Could you check a few things on this model? Use its own coordinates, in mm. Round coordinates to 2 decimals unless told otherwise and drop trailing zeros. Loops run counter-clockwise (first coordinate to the right, second up) from the corner with the lowest first, then second, coordinate; pieces in that order, holes last. Notation, with made-up numbers: (36.5, 39) - (82.5, 39) arc R19 ccw to (82.5, 70) - close; hole circle Ø4 at (74, -32.5). An arc over 180 degrees is marked (long way). Put each result on its own line as item: value. Start each with the question number.
from build123d import *

# Parameters (mm, degrees)
F0_R     = 10
F1_DEPTH = 2.5


with BuildPart() as f1:
    # F0 (on Front) → F1 (new body, symmetric)
    with BuildSketch(Plane.XZ):
        with BuildLine():
            ThreePointArc((0, 15), (10.606602, 10.606602), (15, 0))
            ThreePointArc((15, 0), (10.606602, -10.606602), (0, -15))
            Line((0, -15), (180, -15))
            ThreePointArc((180, -15), (165, 0), (180, 15))
            Line((180, 15), (0, 15))
        make_face()
        with BuildLine():
            ThreePointArc((0, -15), (10.606602, -10.606602), (15, 0))
            ThreePointArc((15, 0), (10.606602, 10.606602), (0, 15))
            ThreePointArc((0, 15), (-15, 0), (0, -15))
        make_face()
        Circle(F0_R, mode=Mode.SUBTRACT)
        with BuildLine():
            ThreePointArc((195, 0), (190.606602, 10.606602), (180, 15))
            ThreePointArc((180, 15), (165, 0), (180, -15))
            ThreePointArc((180, -15), (190.606602, -10.606602), (195, 0))
        make_face()
        with Locations((180, 0)):
            Circle(F0_R, mode=Mode.SUBTRACT)
    extrude(amount=F1_DEPTH, both=True)


solid = f1.part
Item 1: I need wall thicknesses on line 1 (X direction, y = -1.9, z = -7); line 2 (X direction, y = -0.75, z = -3); line 3 (Z direction, x = 0, y = -0.7). Which ranges of each line are inside material? Lowest first, please. Write a range as from..to.
Item 2: Suppose I cut it at C-C, the plane z = 7. List the corners of the cut face in (x, y) for me.
Item 3: Suppose I cut it at B-B, the plane x = 7.5. List the corners of the cut face in (y, z) for me.
Item 4: Will these pins go through, and if not, where does the flat tip stop? P1, Ø1.5, axis at y = -1, z = -11, coming from the +X side; P2, Ø2, axis at y = -1, z = -3, coming from the +X side; P3, Ø16, axis at x = 180, z = 0, coming from the +Y side; P4, Ø1.5, axis at y = -1.5, z = 9, coming from the +X side.
Item 5: Suppose I cut it at A-A, the plane y = 0.5. List the corners of the cut face in (x, z) for me, then the cut area to 3 significant figures.
Item 6: Suppose I cut it at D-D, the plane z = -5. List the corners of the cut face in (x, y) for me, then the cut area to 3 significant figures.
Numbers:
1. line 1: -13.27..-7.14, 7.14..172.86, 187.14..193.27
1. line 2: -14.7..-9.54, 9.54..170.46, 189.54..194.7
1. line 3: -15..-10, 10..15
2. outline: (-13.27, -2.5) - (-7.14, -2.5) - (-7.14, 2.5) - (-13.27, 2.5) - close; (7.14, -2.5) - (172.86, -2.5) - (172.86, 2.5) - (7.14, 2.5) - close; (187.14, -2.5) - (193.27, -2.5) - (193.27, 2.5) - (187.14, 2.5) - close
3. outline: (-2.5, -15) - (2.5, -15) - (2.5, -6.61) - (-2.5, -6.61) - close; (-2.5, 6.61) - (2.5, 6.61) - (2.5, 15) - (-2.5, 15) - close
4. P1: x = 190.95
4. P2: x = 194.87
4. P3: through
4. P4: x = 192.53
5. outline: (0, -15) - (180, -15) arc R15 ccw to (195, 0) arc R15 ccw to (180, 15) - (0, 15) arc R15 ccw to start; hole circle Ø20 at (0, 0); hole circle Ø20 at (180, 0)
5. area: 5,480 mm^2
6. outline: (-14.14, -2.5) - (-8.66, -2.5) - (-8.66, 2.5) - (-14.14, 2.5) - close; (8.66, -2.5) - (171.34, -2.5) - (171.34, 2.5) - (8.66, 2.5) - close; (188.66, -2.5) - (194.14, -2.5) - (194.14, 2.5) - (188.66, 2.5) - close
6. area: 868 mm^2
